Could you check a few things on this drawing? It's one solid part, dimensions in mm from its lowest x, y, z. A direction names the side the tool comes from. Give positions to 0.01 mm unless a question says otherwise; leave off trailing zeros. Loops run counter-clockwise (first coordinate to the right, second up) from the corner with the lowest first, then second, coordinate; pieces in that order, holes last. Notation, with made-up numbers: (82.25, 26.25) - (97.25, 26.25) arc R29 cw to (97.25, 49.25) - close; hole circle Ø10 at (-22, 77.25). An arc over 180 degrees is marked (long way). Write each question's results on one line, items separated by ' | '. Start each with the question number.
(1) Suppose I cut it at A-A (x = 21). Please give me the cut outline in (y, z).
(2) Suppose I cut it at C-C (x = 35). Please give me the cut outline in (y, z), and give its area (3 significant figures).
(3) I need wall thicknesses on line 1 (Y direction, x = 79, z = 2); line 2 (Z direction, x = 5, y = 106.5); line 3 (Y direction, x = 49, z = 38). Which ranges of each line are inside material? Lowest first, please.
(4) On a 3-axis mill with a long thin cutter (end or side, diameter ignored), from which of +Z, -Z, +X, -X, +Y, -Y can I reach the whole of each face in a straight line? I mean the marked faces 1, 2 and 3. Say none if no direction works.
(5) For pin 1 (19.5 mm diameter, centred on y = 40, z = 41.5, fed in from +X); pin 2 (11 mm diameter, centred on x = 50, z = 41, fed in from -Y); pin 3 (4 mm diameter, centred on x = 27, y = 57.5, fed in from +Z), each with a flat end and sliding along its axis, tell me the tip position at first contact or that it passes through.
(6) Suppose I cut it at D-D (z = 13). Please give me the cut outline in (x, y).
(7) Suppose I cut it at B-B (y = 19). Please give me the cut outline in (x, z).
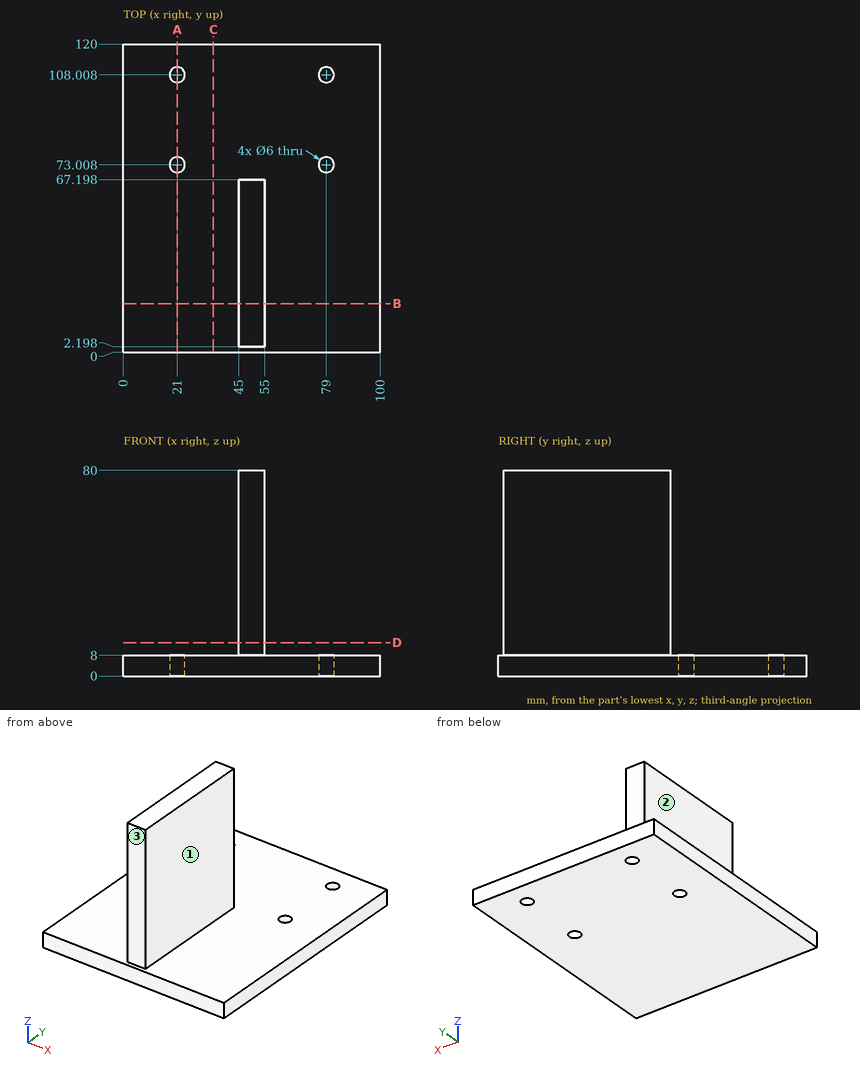
Output values:
1) outline: (0, 0) - (70.01, 0) - (70.01, 8) - (0, 8) - close; (76.01, 0) - (105.01, 0) - (105.01, 8) - (76.01, 8) - close; (111.01, 0) - (120, 0) - (120, 8) - (111.01, 8) - close
2) outline: (0, 0) - (120, 0) - (120, 8) - (0, 8) - close | area: 960 mm2
3) line 1: 0 to 70.01, 76.01 to 105.01, 111.01 to 120 | line 2: 0 to 8 | line 3: 2.2 to 67.2
4) face 1: +Z, +X, +Y, -Y | face 2: +Z, -X, +Y, -Y | face 3: +Z, +X, -X, -Y
5) pin 1: x = 55 | pin 2: y = 2.2 | pin 3: z = 8
6) outline: (45, 2.2) - (55, 2.2) - (55, 67.2) - (45, 67.2) - close
7) outline: (0, 0) - (100, 0) - (100, 8) - (55, 8) - (55, 80) - (45, 80) - (45, 8) - (0, 8) - close
